Source: CAD feature listing. Evaluate the final solid. Frame: model axes, mm. Face numbers are marked on the shaded views. A direction names the side the tool comes from. Round coordinates to 2 decimals unless told otherwise and drop trailing zeros. Order: outer loops, then holes, each group sorted by start corner. A loop starts at its lowest first (then second) coordinate and runs counter-clockwise, first axis right, second up. Notation, with made-up numbers: (29, 12) -> (48, 12) arc R19 ccw to (48, 25) -> close; hole circle Ø1 at (-3, 28). An arc over 180 degrees is marked (long way). Answer as CSV lines item,"result". Start each with the question number.
(1) Section query C-C (z = 23). Output: boundary loops of the cut face in (x, y).
(2) Pull-direction query (Y, two-part tool) for the marked faces 1, 2 and 3; classes: +Y half, -Y half, draft (parallel to the pull), parting line (faces both ways), or undercut.
(3) Contact query for flat-ended pins moving along their axis: P1, Ø7.5, axis at y = 185.5, z = 57, coming from the +X side; P2, Ø7.5, axis at y = 188.5, z = 50, coming from the -X side; P3, Ø20, axis at x = 3.5, y = -181.5, coming from the +Z side. Output: stop coordinate, or through.
(4) Set-up query: the marked faces 4 and 5. Return all of +Z, -Z, +X, -X, +Y, -Y with unobstructed straight access to the full face (end or side cutting, diameter ignored); none if empty.
(5) Section query A-A (y = -44). Output: boundary loops of the cut face in (x, z), plus the area to 3 significant figures.
(6) Line query: line 1 along Y through (x, z) = (-66, 38); line 2 along Y through (x, z) = (-22, 52). Output: solid intervals per line, ascending. Write a range as from..to.
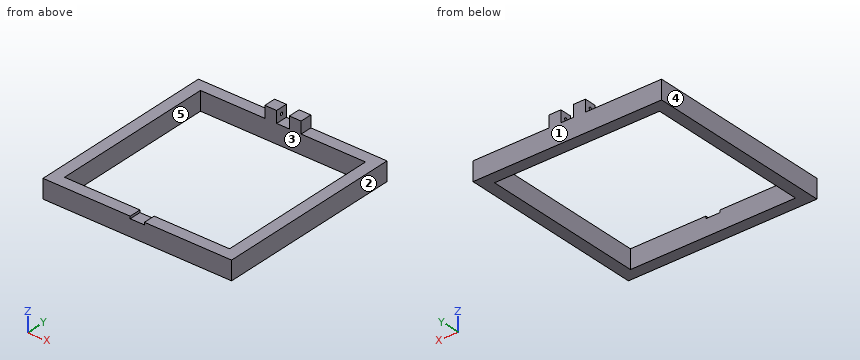
```python
from build123d import *

# Parameters (mm, degrees)
F0_W     = 400
F0_H     = 400
F0_W_2   = 350
F0_H_2   = 350
F1_DEPTH = 40
F2_W     = 30
F2_H     = 5
F3_DEPTH = 25
F4_W     = 25
F4_H     = 25
F5_DEPTH = 25
F6_R     = 3
F7_DEPTH = 5
F8_R     = 3
F9_DEPTH = 25


with BuildPart() as f1:
    # F0 (on Top) → F1 (new body)
    with BuildSketch(Plane.XY):
        Rectangle(F0_W, F0_H)
        Rectangle(F0_W_2, F0_H_2, mode=Mode.SUBTRACT)
    extrude(amount=F1_DEPTH)

    # F2 (on face) → F3 (cut, through all)
    with BuildSketch(Plane.XZ.offset(200)):
        with Locations((0, 37.5)):
            Rectangle(F2_W, F2_H)
    extrude(amount=-F3_DEPTH, mode=Mode.SUBTRACT)

    # F4 (on face) → F5 (join)
    with BuildSketch(Plane.XY.offset(40)):
        with Locations((-26, 187.5)):
            Rectangle(F4_W, F4_H)
        with Locations((26, 187.5)):
            Rectangle(F4_W, F4_H)
    extrude(amount=F5_DEPTH)

    # F6 (on face) → F7 (cut)
    with BuildSketch(Plane(origin=(13.5, 0, 0), x_dir=(0, -1, 0), z_dir=(-1, 0, 0))):
        with Locations((-187.5, 52.5)):
            Circle(F6_R)
    extrude(amount=-F7_DEPTH, mode=Mode.SUBTRACT)

    # F8 (on face) → F9 (cut, through all)
    with BuildSketch(Plane.YZ.offset(-13.5)):
        with Locations((187.5, 52.5)):
            Circle(F8_R)
    extrude(amount=-F9_DEPTH, mode=Mode.SUBTRACT)


solid = f1.part
```
Answer block:
1,outline,"(-200, -200) -> (200, -200) -> (200, 200) -> (-200, 200) -> close; hole (-175, -175) -> (175, -175) -> (175, 175) -> (-175, 175) -> close"
2,face 1,"+Y half"
2,face 2,"draft"
2,face 3,"undercut"
3,P1,"x = 38.5"
3,P2,"x = -38.5"
3,P3,"z = 35"
4,face 4,"+Z, -Z, -X, +Y, -Y"
4,face 5,"+Z, -Z"
5,outline,"(-200, 0) -> (-175, 0) -> (-175, 40) -> (-200, 40) -> close; (175, 0) -> (200, 0) -> (200, 40) -> (175, 40) -> close"
5,area,"2,000 mm2"
6,line 1,"-200..-175, 175..200"
6,line 2,"175..184.54, 190.46..200"
